Part model, mm, in its own coordinate system. Round coordinates to 2 decimals unless told otherwise and drop trailing zeros. Write each loop counter-clockwise with the first axis right and the second up, starting at its lowest first coordinate (ties: lowest second). Pieces come first, ordered by that corner, then holes. Notation, with made-up numbers: M 55,15 L 72,15 A31 cw 72,48 Z; hole C 80,-2.5 d5. An arc over 180 degrees is marked long. Use one line per item in the form item = value. Start each with the question number.
Item 1: Probe L1, parallel to X at y = 437, z = 1.1; L2, parallel to X at y = 421, z = 0.4; L3, parallel to X at y = 431.5, z = 0.55. List the from-to ranges inside material, lowest first.
Item 2: Cut at B-B, the plane x = 583.5. Give the cut face in (y, z), then the cut area to 3 significant figures.
Item 3: Cut at A-A, the plane y = 418.5. Give the cut face in (x, z).
Item 4: Cut at D-D, the plane x = 574.5. Give the cut face in (y, z).
Item 5: Cut at C-C, the plane y = 445. Give the cut face in (x, z), then the cut area to 3 significant figures.
Item 6: Flat gauge pins, fed straight in: pin 1 Ø1 at (x, y) = (595.5, 438) entering from -Z; pin 2 Ø3 at (x, y) = (564.76, 402.97) entering from +Z; pin 3 Ø0.8 at (x, z) = (585, 1) entering from -Y. Where does each tip first touch, or does it go through?
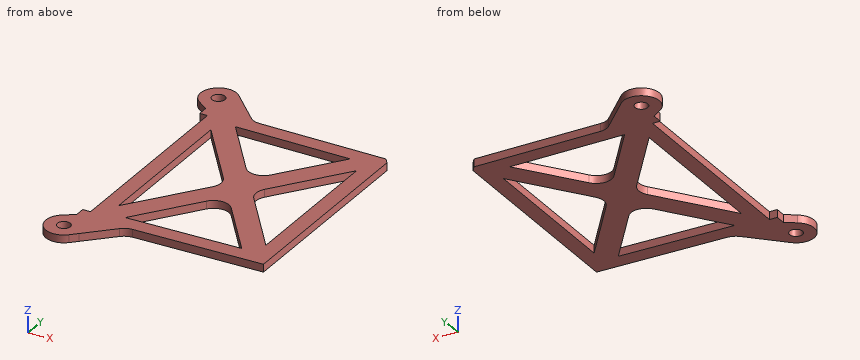
from build123d import *

# Parameters (mm, degrees)
MODEL_R         = 1.25
EXTRUDE_2_DEPTH = 1.5


with BuildPart() as part:
    # Model → 凸台-拉伸2 (new body)
    with BuildSketch(Plane.XY):
        with BuildLine():
            Line((567.23508643, 456.796470283), (573.081278388, 450.950276374))
            ThreePointArc((573.081278388, 450.950276374), (574.054548435, 450.29995812), (575.202598732, 450.071596717))
            Line((575.202598732, 450.071596717), (599.702598732, 450.071596717))
            Line((599.702598732, 450.071596717), (600.534867908, 449.022451897))
            Line((600.534867908, 449.022451897), (600.534867908, 408.022451897))
            Line((600.534867908, 408.022451897), (575.481922704, 407.463178676))
            ThreePointArc((575.481922704, 407.463178676), (574.371365784, 407.209391557), (573.427556635, 406.571450445))
            Line((573.427556635, 406.571450445), (568.455496448, 401.695722345))
            Line((568.455496448, 401.695722345), (567.235086299, 400.498957255))
            ThreePointArc((567.235086299, 400.498957255), (562.070444361, 400.734378517), (562.774755691, 405.856184357))
            Line((562.774755691, 405.856184357), (564.760216971, 407.22383333))
            Line((564.760216971, 407.22383333), (564.760216971, 409.22383333))
            Line((564.760216971, 409.22383333), (566.260216971, 409.22383333))
            Line((566.260216971, 409.22383333), (566.260216971, 448.071599095))
            Line((566.260216971, 448.071599095), (564.760216971, 448.071599095))
            Line((564.760216971, 448.071599095), (564.760216971, 450.071599095))
            Line((564.760216971, 450.071599095), (562.774760372, 451.439240088))
            ThreePointArc((562.774760372, 451.439240088), (562.070442602, 456.56104704), (567.23508643, 456.796470283))
        make_face()
        with Locations((564.760212527, 454.321596717)):
            Circle(MODEL_R, mode=Mode.SUBTRACT)
        with Locations((564.760212527, 402.973830952)):
            Circle(MODEL_R, mode=Mode.SUBTRACT)
        with BuildLine():
            ThreePointArc((579.517792138, 427.066754763), (580.118537337, 428.881766433), (579.50090837, 430.691102394))
            Line((579.50090837, 430.691102394), (569.260212527, 444.071596717))
            Line((569.260212527, 444.071596717), (569.260212527, 413.402282802))
            Line((569.260212527, 413.402282802), (579.517792138, 427.066754763))
        make_face(mode=Mode.SUBTRACT)
        with BuildLine():
            ThreePointArc((581.084435265, 435.507954993), (583.481204613, 434.327912105), (585.868577071, 435.526852168))
            Line((585.868577071, 435.526852168), (594.534929977, 447.071596717))
            Line((594.534929977, 447.071596717), (572.260212527, 447.071596717))
            Line((572.260212527, 447.071596717), (581.084435265, 435.507954993))
        make_face(mode=Mode.SUBTRACT)
        with BuildLine():
            ThreePointArc((585.96375898, 422.246741072), (583.565361337, 423.423386992), (581.179698264, 422.221131371))
            Line((581.179698264, 422.221131371), (572.333907172, 410.403188089))
            Line((572.333907172, 410.403188089), (594.609247843, 410.950544366))
            Line((594.609247843, 410.950544366), (585.96375898, 422.246741072))
        make_face(mode=Mode.SUBTRACT)
        with BuildLine():
            ThreePointArc((587.511830306, 430.680835717), (586.913584899, 428.869200497), (587.528632984, 427.063200611))
            Line((587.528632984, 427.063200611), (597.535553197, 413.949701149))
            Line((597.535553197, 413.949701149), (597.534929977, 444.071658787))
            Line((597.534929977, 444.071658787), (587.511830306, 430.680835717))
        make_face(mode=Mode.SUBTRACT)
    extrude(amount=EXTRUDE_2_DEPTH)


solid = part.part
Model answer:
q1.L1 = 566.26 to 569.26, 574.67 to 579.95, 586.97 to 592.24, 597.54 to 600.53
q1.L2 = 566.26 to 569.26, 574.96 to 580.27, 586.92 to 592.16, 597.54 to 600.53
q1.L3 = 566.26 to 569.26, 578.88 to 588.12, 597.54 to 600.53
q2.outline = M 407.64,0 L 410.68,0 L 410.68,1.5 L 407.64,1.5 Z; M 423.42,0 L 434.33,0 L 434.33,1.5 L 423.42,1.5 Z; M 447.07,0 L 450.07,0 L 450.07,1.5 L 447.07,1.5 Z
q2.area = 25.4 mm²
q3.outline = M 566.26,0 L 569.26,0 L 569.26,1.5 L 566.26,1.5 Z; M 573.09,0 L 578.39,0 L 578.39,1.5 L 573.09,1.5 Z; M 588.83,0 L 594.06,0 L 594.06,1.5 L 588.83,1.5 Z; M 597.54,0 L 600.53,0 L 600.53,1.5 L 597.54,1.5 Z
q4.outline = M 407.26,0 L 410.46,0 L 410.46,1.5 L 407.26,1.5 Z; M 413.3,0 L 420.38,0 L 420.38,1.5 L 413.3,1.5 Z; M 437.23,0 L 444.14,0 L 444.14,1.5 L 437.23,1.5 Z; M 447.07,0 L 450.16,0 L 450.16,1.5 L 447.07,1.5 Z
q5.outline = M 566.26,0 L 573.84,0 L 573.84,1.5 L 566.26,1.5 Z; M 592.98,0 L 600.53,0 L 600.53,1.5 L 592.98,1.5 Z
q5.area = 22.7 mm²
q6.pin_1 = through
q6.pin_2 = 1.5
q6.pin_3 = 407.67
